Read the model definition and answer for the solid it produces. Units are mm, in the model's axes. Face numbers are marked on the shaded views. A direction names the side the tool comes from. Coordinates: 2 decimals unless noted, no trailing zeros. Write each loop counter-clockwise with the first axis right and the second up, starting at its lowest first coordinate (ties: lowest second). Pieces come first, ordered by that corner, then holes.
(1) Straight lines are drawn through the part: line 1 along X through (y, z) = (-13.5, 0); line 2 along X through (y, z) = (-7, 0); line 3 along Z through (x, y) = (18, -1). For each, find the intervals that lie inside material, in ascending order.
(2) Which of the six approach directions +Z, -Z, +X, -X, +Y, -Y give full straight-line access (tool end or side, diameter ignored) to the marked faces 4 and 5?
(3) The part is cut by section D-D, the plane x = 259.5. Determine the outline of the cut face in (y, z).
(4) Determine the mould class of the marked faces 1, 2 and 3 for opening direction Z: pulls with the +Z half, pulls with the -Z half, needs draft (parallel to the pull), parting line crosses it, or undercut.
(5) The part is cut by section C-C, the plane x = 18. Determine the outline of the cut face in (y, z), and give its area (3 significant figures).
(6) The part is cut by section B-B, the plane y = 0. Determine the outline of the cut face in (x, z).
(7) Given pin 1 (1 mm diameter, centred on y = -17.5, z = 4, fed in from +X); pin 2 (6 mm diameter, centred on x = 98.5, z = -4, fed in from +Y); pin 3 (4 mm diameter, centred on x = 81, z = -15, fed in from -Y), each flat-ended and moving along its own axis, determine where each tip first touches the part or whether it passes through.
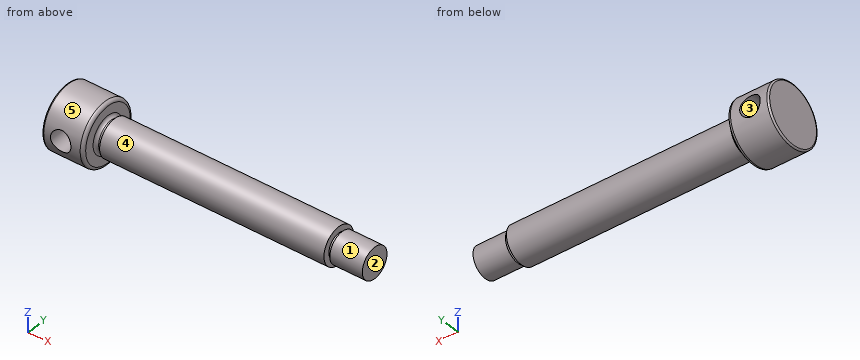
```python
from build123d import *

# Parameters (mm, degrees)
FILLET1_R               = 1.5
CUT_EXTRUDE1_DEPTH      = 303.985148161
CUT_EXTRUDE1_DEPTH_BACK = 303.985148161
SKETCH2_R               = 10
FILLET2_R               = 3


with BuildPart() as part:
    # Sketch1 → Revolve1 (revolve)
    with BuildSketch(Plane.XY, mode=Mode.PRIVATE) as revolve1_sk:
        Polygon((0, 0), (0, 30), (40, 30), (40, 15), (46.35, 15), (46.35, 18), (265, 18), (265, 12), (268.35, 12), (268.35, 15), (300, 15), (300, 0), align=None)
    revolve(revolve1_sk.sketch.rotate(Axis((0, 0, 0), (1, 0, 0)), 90), axis=Axis((0, 0, 0), (1, 0, 0)))

    # Fillet1
    fillet1_edges = [part.edges().sort_by_distance(p)[0] for p in [
        (0, 0, -30),
    ]]
    fillet(fillet1_edges, radius=FILLET1_R)

    # Sketch2 → Cut-Extrude1 (cut, two sides: drawn at the far end of the back side and taken through both)
    with BuildSketch(Plane(origin=(0, 0, 0), x_dir=(1, 0, 0), z_dir=(0, 1, 0)).offset(-CUT_EXTRUDE1_DEPTH_BACK)):
        with Locations(Location((18, 0, 0), (0, 0, 270))):
            Circle(SKETCH2_R)
    extrude(amount=CUT_EXTRUDE1_DEPTH + CUT_EXTRUDE1_DEPTH_BACK, mode=Mode.SUBTRACT)

    # Fillet2
    fillet2_edges = [part.edges().sort_by_distance(p)[0] for p in [
        (40, 0, -15),
        (40, 0, -30),
    ]]
    fillet(fillet2_edges, radius=FILLET2_R)


solid = part.part
```
Computed:
1. line 1: x = 0 to 8, 28 to 265, 268.35 to 300
1. line 2: x = 0 to 8, 28 to 300
1. line 3: z = -29.98 to -10, 10 to 29.98
2. face 4: +X
2. face 5: +X, -X
3. outline: circle Ø36 at (0, 0)
4. face 1: parting line crosses it
4. face 2: needs draft
4. face 3: undercut
5. outline: (-28.28, -10) arc R30 ccw to (28.28, -10) - close; (-28.28, 10) - (28.28, 10) arc R30 ccw to start
5. area: 1,650 mm2
6. outline: (0, -28.5) arc R1.5 ccw to (1.5, -30) - (37, -30) arc R3 ccw to (40, -27) - (40, -18) arc R3 cw to (43, -15) - (46.35, -15) - (46.35, -18) - (265, -18) - (265, -12) - (268.35, -12) - (268.35, -15) - (300, -15) - (300, 15) - (268.35, 15) - (268.35, 12) - (265, 12) - (265, 18) - (46.35, 18) - (46.35, 15) - (43, 15) arc R3 cw to (40, 18) - (40, 27) arc R3 ccw to (37, 30) - (1.5, 30) arc R1.5 ccw to (0, 28.5) - close; hole circle Ø20 at (18, 0)
7. pin 1: stops at x = 265
7. pin 2: stops at y = 17.97
7. pin 3: stops at y = -12.45
